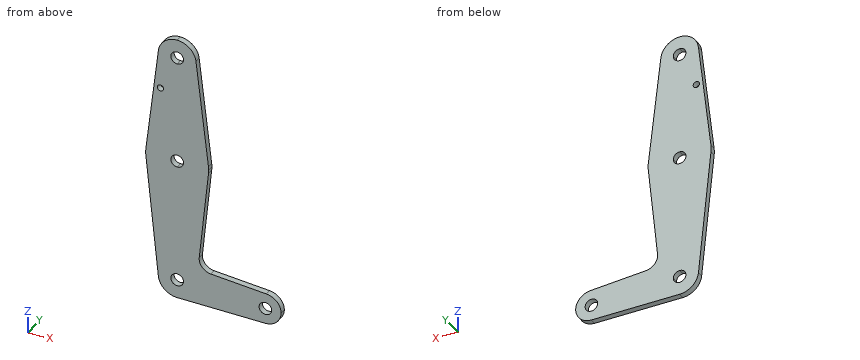
```python
from build123d import *

# Parameters (mm, degrees)
F0_R     = 1.5875
F0_R_2   = 3.175
F1_DEPTH = 3.048


with BuildPart() as f1:
    # F0 (on Front) → F1 (new body)
    with BuildSketch(Plane.XZ):
        with BuildLine():
            ThreePointArc((0, 55.163064), (2.245064, 54.233128), (3.175, 51.988064))
            ThreePointArc((3.175, 51.988064), (2.245064, 49.743), (0, 48.813064))
            Line((0, 48.813064), (0, 42.463064))
            ThreePointArc((0, 42.463064), (6.735192, 45.252872), (9.525, 51.988064))
            ThreePointArc((9.525, 51.988064), (9.509147, 52.537388), (9.461639, 53.084883))
            ThreePointArc((9.461639, 53.084883), (6.335551, 59.100477), (0, 61.513064))
            Line((0, 61.513064), (0, 55.163064))
        make_face()
        with BuildLine():
            ThreePointArc((0, 48.813064), (-3.175, 51.988064), (0, 55.163064))
            Line((0, 55.163064), (0, 61.513064))
            ThreePointArc((0, 61.513064), (-6.335551, 59.100477), (-9.461639, 53.084883))
            ThreePointArc((-9.461639, 53.084883), (-7.112413, 45.652513), (0, 42.463064))
            Line((0, 42.463064), (0, 48.813064))
        make_face()
        with BuildLine():
            Line((0, 12.718398), (0, 42.463064))
            ThreePointArc((0, 42.463064), (-7.112413, 45.652513), (-9.461639, 53.084883))
            Line((-9.461639, 53.084883), (-15.769398, -1.32857))
            ThreePointArc((-15.769398, -1.32857), (-10.559252, 8.697419), (0, 12.718398))
        make_face()
        with Locations((-8.408644, 33.368598)):
            Circle(F0_R, mode=Mode.SUBTRACT)
        with BuildLine():
            ThreePointArc((9.525, 51.988064), (6.735192, 45.252872), (0, 42.463064))
            Line((0, 42.463064), (0, 12.718398))
            ThreePointArc((0, 12.718398), (10.559252, 8.697419), (15.769398, -1.32857))
            Line((15.769398, -1.32857), (9.461639, 53.084883))
            ThreePointArc((9.461639, 53.084883), (9.509147, 52.537388), (9.525, 51.988064))
        make_face()
        with BuildLine():
            Line((0, 0.018398), (0, 12.718398))
            ThreePointArc((0, 12.718398), (-10.559252, 8.697419), (-15.769398, -1.32857))
            ThreePointArc((-15.769398, -1.32857), (-15.874539, -3.035634), (-15.795426, -4.744102))
            ThreePointArc((-15.795426, -4.744102), (-10.649274, -14.929817), (0, -19.031602))
            Line((0, -19.031602), (0, -6.331602))
            ThreePointArc((0, -6.331602), (-3.175, -3.156602), (0, 0.018398))
        make_face()
        with BuildLine():
            ThreePointArc((15.769398, -1.32857), (10.559252, 8.697419), (0, 12.718398))
            Line((0, 12.718398), (0, 0.018398))
            ThreePointArc((0, 0.018398), (2.245064, -0.911538), (3.175, -3.156602))
            ThreePointArc((3.175, -3.156602), (2.245064, -5.401666), (0, -6.331602))
            Line((0, -6.331602), (0, -19.031602))
            ThreePointArc((0, -19.031602), (10.649274, -14.929817), (15.795426, -4.744102))
            ThreePointArc((15.795426, -4.744102), (15.855094, -3.951349), (15.875, -3.156602))
            ThreePointArc((15.875, -3.156602), (15.848578, -2.241062), (15.769398, -1.32857))
        make_face()
        with BuildLine():
            ThreePointArc((0, -19.031602), (-10.649274, -14.929817), (-15.795426, -4.744102))
            Line((-15.795426, -4.744102), (-9.477255, -67.609102))
            ThreePointArc((-9.477255, -67.609102), (-7.063929, -60.267038), (0, -57.131602))
            Line((0, -57.131602), (0, -19.031602))
        make_face()
        with BuildLine():
            Line((11.111022, -51.353331), (15.795426, -4.744102))
            ThreePointArc((15.795426, -4.744102), (10.649274, -14.929817), (0, -19.031602))
            Line((0, -19.031602), (0, -57.131602))
            ThreePointArc((0, -57.131602), (6.735192, -59.92141), (9.525, -66.656602))
            ThreePointArc((9.525, -66.656602), (6.735192, -73.391794), (0, -76.181602))
            Line((0, -76.181602), (44.421643, -76.181602))
            ThreePointArc((44.421643, -76.181602), (36.489207, -67.96062), (44.988245, -60.326851))
            Line((44.988245, -60.326851), (16.97591, -58.322132))
            ThreePointArc((16.97591, -58.322132), (12.570778, -56.077134), (11.111022, -51.353331))
        make_face()
        with BuildLine():
            ThreePointArc((3.175, -66.656602), (2.245064, -64.411538), (0, -63.481602))
            ThreePointArc((0, -63.481602), (-2.245064, -68.901666), (3.175, -66.656602))
        make_face()
        with BuildLine():
            ThreePointArc((0, -57.131602), (-7.063929, -60.267038), (-9.477255, -67.609102))
            ThreePointArc((-9.477255, -67.609102), (-6.389564, -73.720531), (0, -76.181602))
            ThreePointArc((0, -76.181602), (6.735192, -73.391794), (9.525, -66.656602))
            ThreePointArc((9.525, -66.656602), (6.735192, -59.92141), (0, -57.131602))
        make_face()
        with BuildLine():
            ThreePointArc((3.175, -66.656602), (-2.245064, -68.901666), (0, -63.481602))
            ThreePointArc((0, -63.481602), (2.245064, -64.411538), (3.175, -66.656602))
        make_face(mode=Mode.SUBTRACT)
        with BuildLine():
            ThreePointArc((44.988245, -60.326851), (36.489207, -67.96062), (44.421643, -76.181602))
            ThreePointArc((44.421643, -76.181602), (50.034303, -73.856762), (52.359143, -68.244102))
            ThreePointArc((52.359143, -68.244102), (50.231174, -62.835475), (44.988245, -60.326851))
        make_face()
        with Locations((44.421643, -68.244102)):
            Circle(F0_R_2, mode=Mode.SUBTRACT)
    extrude(amount=F1_DEPTH)


solid = f1.part
```
Input: part model. Units: mm. Frame: model coordinates. Coordinates: 2 decimals unless noted, no trailing zeros. Order: outer loops, then holes, each group sorted by start corner. A loop starts at its lowest first (then second) coordinate and runs counter-clockwise, first axis right, second up. Notation, with made-up numbers: (-8.75, 19.25) - (2.25, 19.25) arc R11 ccw to (2.25, 32.25) - close; hole circle Ø5 at (-38.5, 46.5). An arc over 180 degrees is marked (long way). Put each result on its own line as item: value.
1. Cut plane A-A on y = -2.55. State how many separate pieces and enclosed holes the cut face has, then the cut area to 3 significant figures.
Report:
separate pieces: 1
enclosed holes: 5
area: 3,900 mm2
2. Cut plane C-C on z = -12.5. Return the cut outline in (x, y), then the cut area to 3 significant figures.
Report:
outline: (-15.02, -3.05) - (15.02, -3.05) - (15.02, 0) - (-15.02, 0) - close
area: 91.5 mm2
3. Line query: line 1 along Z through (x, y) = (0.5, -2.85); line 2 along Z through (x, y) = (42, -0.85); line 3 along X through (y, z) = (-2.45, -65). Output: solid intervals per line, ascending.
Report:
line 1: z = -76.18 to -69.79, -63.52 to -6.29, -0.02 to 48.85, 55.12 to 61.5
line 2: z = -76.18 to -70.3, -66.19 to -60.11
line 3: x = -9.74 to -2.71, 2.71 to 51.67
4. Cut plane B-B on x = 29. Return the cut outline in (y, z), then the cut area to 3 significant figures.
Report:
outline: (-3.05, -76.18) - (0, -76.18) - (0, -59.18) - (-3.05, -59.18) - close
area: 51.8 mm2
5. Contact query for a flat-ended pin moving along its axis: pin 1 Ø1.5 at (y, z) = (-0.5, -59.5) entering from -X. Output: stop coordinate, or through.
Report:
pin 1: stops at x = -10.37
